from build123d import *

# Parameters (mm, degrees)
SKETCH1_W           = 63
SKETCH1_H           = 45
BOSS_EXTRUDE1_DEPTH = 23
CUT_EXTRUDE1_DEPTH  = 18


with BuildPart() as part:
    # Sketch1 → Boss-Extrude1 (new body)
    with BuildSketch(Plane(origin=(0, 0, 0), x_dir=(1, 0, 0), z_dir=(0, 1, 0))):
        Rectangle(SKETCH1_W, SKETCH1_H)
    extrude(amount=BOSS_EXTRUDE1_DEPTH)

    # Sketch2 → Cut-Extrude1 (cut)
    with BuildSketch(Plane(origin=(0, 23, 0), x_dir=(1, 0, 0), z_dir=(0, 1, 0))):
        with BuildLine():
            Line((24, 5), (38.956997059, 5))
            ThreePointArc((38.956997059, 5), (43.956997059, 0), (38.956997059, -5))
            Line((38.956997059, -5), (24, -5))
            ThreePointArc((24, -5), (19, 0), (24, 5))
        make_face()
        with BuildLine():
            Line((-24, 5), (-38.956997059, 5))
            ThreePointArc((-38.956997059, 5), (-43.956997059, 0), (-38.956997059, -5))
            Line((-38.956997059, -5), (-24, -5))
            ThreePointArc((-24, -5), (-19, 0), (-24, 5))
        make_face()
    extrude(amount=-CUT_EXTRUDE1_DEPTH, mode=Mode.SUBTRACT)


solid = part.part
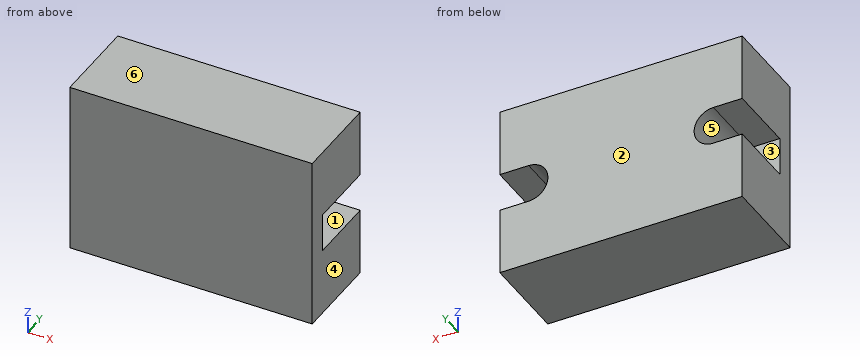
The listing builds one solid part. Answer for the finished solid, in the listing's coordinates (mm). Face numbers are marked on the shaded views. A direction names the side the tool comes from. Round coordinates to 2 decimals unless told otherwise and drop trailing zeros. Order: outer loops, then holes, each group sorted by start corner. A loop starts at its lowest first (then second) coordinate and runs counter-clockwise, first axis right, second up. Notation, with made-up numbers: (67.5, 47) - (87.5, 47) arc R7 cw to (87.5, 52) - close; hole circle Ø5 at (-27.75, 61). An arc over 180 degrees is marked (long way). Write item = value, one per line. Start each with the question number.
1) Section A-A, the plane x = -20 is taken. Write down the section's boundary in (y, z), plus the area to 3 significant figures.
2) Straight lines are drawn through the part: L1, parallel to Z at x = 26.5, y = 21.75; L2, parallel to Y at x = 24, z = -2.5; L3, parallel to X at y = 18.5, z = 0. For each, find the intervals that lie inside material, in ascending order.
3) Given pin 1 (11 mm diameter, centred on x = 23, z = 2, fed in from +Y); pin 2 (8 mm diameter, centred on x = -28, z = 0.5, fed in from +Y), each flat-ended and moving along its own axis, determine where each tip first touches the part or whether it passes through.
4) Section C-C, the plane z = 0 is taken. Write down the section's boundary in (x, y), plus the area to 3 significant figures.
5) For the marked faces 1, 2 and 3, determine the directions among +Z, -Z, +X, -X, +Y, -Y from which every point of the face is accessible in a straight line to the end or side of a thin tool.
6) For a pull along Z with two mould halves and no side action, classify the marked faces 4, 5 and 6 as released by +Z, released by -Z, zero draft, split by the parting line, or undercut.
7) Section B-B, the plane y = 16.25 is taken. Write down the section's boundary in (x, z), plus the area to 3 significant figures.
Results list:
q1.outline = (0, -22.5) - (23, -22.5) - (23, -3) - (5, -3) - (5, 3) - (23, 3) - (23, 22.5) - (0, 22.5) - close
q1.area = 927 mm^2
q2.L1 = -22.5 to -5, 5 to 22.5
q2.L2 = 0 to 5
q2.L3 = -19 to 19
q3.pin_1 = 23
q3.pin_2 = 5
q4.outline = (-31.5, 0) - (31.5, 0) - (31.5, 5) - (19, 5) - (19, 23) - (-19, 23) - (-19, 5) - (-31.5, 5) - close
q4.area = 999 mm^2
q5.face_1 = +X, +Y
q5.face_2 = +Z, -Z, +X, -X, +Y
q5.face_3 = -X, +Y
q6.face_4 = zero draft
q6.face_5 = undercut
q6.face_6 = released by +Z
q7.outline = (-31.5, -22.5) - (31.5, -22.5) - (31.5, -5) - (24, -5) arc R5 cw to (24, 5) - (31.5, 5) - (31.5, 22.5) - (-31.5, 22.5) - (-31.5, 5) - (-24, 5) arc R5 cw to (-24, -5) - (-31.5, -5) - close
q7.area = 2,610 mm^2
